from build123d import *

# Parameters (mm, degrees)
SKETCH1_R                   = 25.4
BOSS_EXTRUDE1_DEPTH         = 10
TAP_DRILL_FOR_M6X1_0_TAP1_D = 5
CIRPATTERN1_COUNT           = 4
SKETCH3_R                   = 7.5
BOSS_EXTRUDE2_DEPTH         = 53.27
SKETCH12_W                  = 1.5
SKETCH12_H                  = 1


with BuildPart() as part:
    # Sketch1 → Boss-Extrude1 (new body)
    with BuildSketch(Plane.XY):
        Circle(SKETCH1_R)
    extrude(amount=BOSS_EXTRUDE1_DEPTH)

    # Tap Drill for M6x1.0 Tap1 (through all)
    with Locations(Plane.XY.offset(10)):
        with Locations((0, 15)):
            tap_drill_for_m6x1_0_tap1 = Hole(TAP_DRILL_FOR_M6X1_0_TAP1_D / 2)

    # CirPattern1: Tap Drill for M6x1.0 Tap1 ×4 about axis
    cirpattern1_axis = Axis((0, 0, 0), (0, 0, 1))
    for i in range(1, CIRPATTERN1_COUNT):
        add(tap_drill_for_m6x1_0_tap1.rotate(cirpattern1_axis, i * 360 / CIRPATTERN1_COUNT), mode=Mode.SUBTRACT)

    # Sketch3 → Boss-Extrude2 (add)
    with BuildSketch(Plane.XY.offset(10)):
        with Locations(Location((0, 0, 0), (0, 0, 180))):
            Circle(SKETCH3_R)
    extrude(amount=BOSS_EXTRUDE2_DEPTH)

    # Sketch12 → Cut-Revolve2 (revolve, cut)
    with BuildSketch(Plane(origin=(0, 0, 0), x_dir=(1, 0, 0), z_dir=(0, 1, 0))):
        with Locations((-7.5, -57.09)):
            Rectangle(SKETCH12_W, SKETCH12_H)
    revolve(axis=Axis((0, 0, 63.27), (0, 0, -1)), mode=Mode.SUBTRACT)


solid = part.part
Here's how the part is built. I have some questions about the finished solid (model axes, mm). A direction names the side the tool comes from. Coordinates: 2 decimals unless noted, no trailing zeros. Loops run counter-clockwise (first coordinate to the right, second up) from the corner with the lowest first, then second, coordinate; pieces in that order, holes last.
1. I need wall thicknesses on L1, parallel to Y at x = 0, z = 6.25; L2, parallel to Z at x = -7.5, y = 15.5; L3, parallel to X at y = -17, z = 5. Which ranges of each line are inside material? Lowest first, please.
2. If we mould it in two halves opening along Z, with no side actions, what happens to faces 1 (the cylindrical face through (-12.56, 0.54, 4.93)), 2 (the flat face through (5, 6, 10)), 3 (the flat face through (7, 1, 56.59))? For each: pulls with the +Z half, pulls with the -Z half, needs draft (parallel to the pull), parting line crosses it, or undercut.
3. For faces 4 (the cylindrical face through (-4.032, -6.324, 32.969)), 5 (the flat face through (0, 0, 63.27)), 6 (the cylindrical face through (1.46, -6.59, 57.08)), which set-ups out of +Z, -Z, +X, -X, +Y, -Y let a thin tool reach every point of the face, with its end or its side?
4. Imagine slicing it at C-C, the plane y = 15. Please give me the cut outline in (x, z).
5. For P1, Ø3, axis at y = 0, z = 43.5, coming from the +X side; P2, Ø1, axis at x = 11, y = -18.5, coming from the +Z side; P3, Ø10, axis at y = -11, z = 36, coming from the -X side; P4, Ø4.5, axis at x = -2, y = -1, coming from the -Z side, each with a flat end and sliding along its axis, tell me the tip position at first contact or that it passes through.
6. Imagine slicing it at A-A, the plane x = 0. Please give me the cut outline in (y, z), and give its area (3 significant figures).
Taken from the geometry:
1. L1: y = -25.4 to -17.5, -12.5 to 12.5, 17.5 to 25.4
1. L2: z = 0 to 10
1. L3: x = -18.87 to -1.5, 1.5 to 18.87
2. face 1: needs draft
2. face 2: pulls with the +Z half
2. face 3: undercut
3. face 4: +Z
3. face 5: +Z, +X, -X, +Y, -Y
3. face 6: none
4. outline: (-20.5, 0) - (-2.5, 0) - (-2.5, 10) - (-20.5, 10) - close; (2.5, 0) - (20.5, 0) - (20.5, 10) - (2.5, 10) - close
5. P1: stops at x = 7.5
5. P2: stops at z = 10
5. P3: stops at x = -4.5
5. P4: stops at z = 0
6. outline: (-25.4, 0) - (-17.5, 0) - (-17.5, 10) - (-25.4, 10) - close; (-12.5, 0) - (12.5, 0) - (12.5, 10) - (7.5, 10) - (7.5, 56.59) - (6.75, 56.59) - (6.75, 57.59) - (7.5, 57.59) - (7.5, 63.27) - (-7.5, 63.27) - (-7.5, 57.59) - (-6.75, 57.59) - (-6.75, 56.59) - (-7.5, 56.59) - (-7.5, 10) - (-12.5, 10) - close; (17.5, 0) - (25.4, 0) - (25.4, 10) - (17.5, 10) - close
6. area: 1,210 mm2
